For this review, use the dimensioned drawing (mm, ordinates from the lowest corner) and the shaded views. A direction names the side the tool comes from. Round coordinates to 2 decimals unless told otherwise and drop trailing zeros. Write each loop counter-clockwise with the first axis right and the second up, starting at its lowest first coordinate (ties: lowest second). Pieces come first, ordered by that corner, then holes. Notation, with made-up numbers: M -14,30 L 1,30 A14 cw 1,41 Z; hole C -21,-23 d9. An arc over 180 degrees is marked long. Answer in a Markdown table with one row per item.
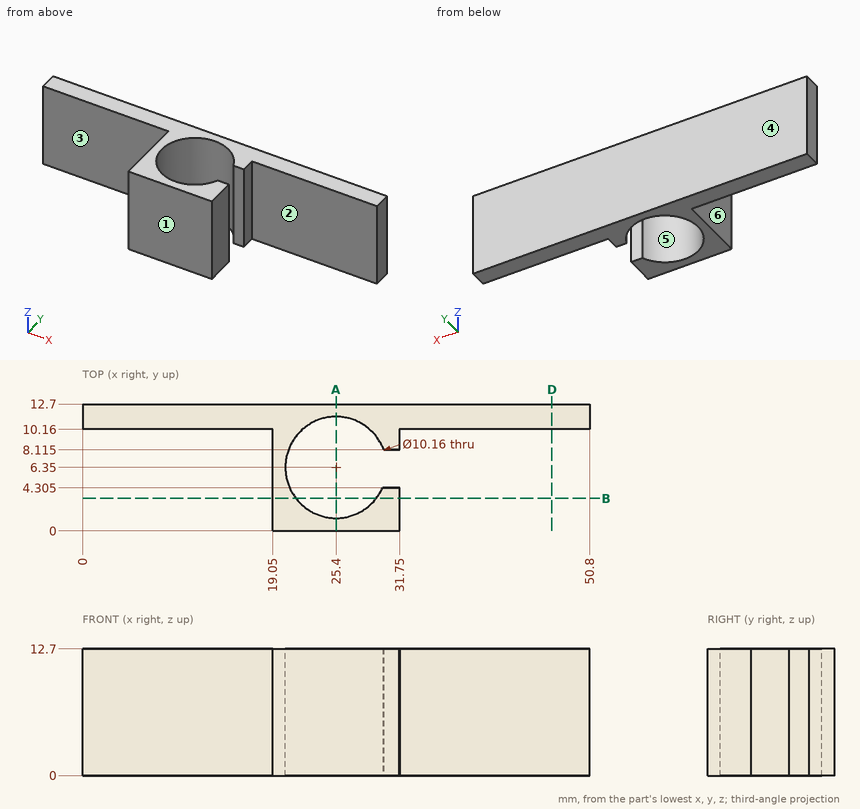
Q1. Machinability: for the marked faces 1, 2 and 3, which of the approach directions +Z, -Z, +X, -X, +Y, -Y give a long, thin tool a straight path to every point of the face, cutting with its end or side? Answer none if there is none.
Found:
| item | result |
|---|---|
| face 1 | +Z, -Z, +X, -X, -Y |
| face 2 | +Z, -Z, +X, -Y |
| face 3 | +Z, -Z, -X, -Y |
Q2. Take a section at D-D (x = 47). State the section outline as (y, z) points, then the cut area to 3 significant figures.
Found:
| item | result |
|---|---|
| outline | M 10.16,0 L 12.7,0 L 12.7,12.7 L 10.16,12.7 Z |
| area | 32.3 mm² |
Q3. Mouldability with a two-part tool opening along Y and no side actions: class the marked faces 4, 5 and 6 as +Y half, -Y half, draft (parallel to the pull), parting line (faces both ways), or undercut.
Found:
| item | result |
|---|---|
| face 4 | +Y half |
| face 5 | undercut |
| face 6 | draft |
Q4. For probe 1 along Y at (x, z) = (25.4, 4.75); probe 2 along Y at (x, z) = (48.5, 5.75); probe 3 along X at (y, z) = (10.5, 1.25), list the stretches that pass through material, from the lowest coordinate up.
Found:
| item | result |
|---|---|
| probe 1 | 0 to 1.27, 11.43 to 12.7 |
| probe 2 | 10.16 to 12.7 |
| probe 3 | 0 to 22.47, 28.33 to 50.8 |
Q5. Insertion check: P1, Ø1.7, axis at x = 30.5, z = 5, coming from the -Y side; P2, Ø6, axis at y = 3.5, z = 7.5, coming from the +X side; P3, Ø6, axis at x = 25.4, y = 6.35, coming from the -Z side; P4, Ø4, axis at x = 7, z = 8.5, coming from the -Y side. Each pin has a flat end and moves straight along its axis. Give the tip position at first contact, or say it passes through.
Found:
| item | result |
|---|---|
| P1 | y = 0 |
| P2 | x = 31.75 |
| P3 | through |
| P4 | y = 10.16 |
Q6. Take a section at B-B (y = 3.25). State the section outline as (x, z) points.
Found:
| item | result |
|---|---|
| outline | M 19.05,0 L 21.38,0 L 21.38,12.7 L 19.05,12.7 Z; M 29.42,0 L 31.75,0 L 31.75,12.7 L 29.42,12.7 Z |
Q7. Take a section at A-A (x = 25.4). State the section outline as (y, z) points.
Found:
| item | result |
|---|---|
| outline | M 0,0 L 1.27,0 L 1.27,12.7 L 0,12.7 Z; M 11.43,0 L 12.7,0 L 12.7,12.7 L 11.43,12.7 Z |
